```python
from build123d import *

# Parameters (mm, degrees)
SKETCH1_W           = 10
SKETCH1_H           = 5
BOSS_EXTRUDE1_DEPTH = 200
SKETCH2_R           = 2.38125
CUT_EXTRUDE1_DEPTH  = 200


with BuildPart() as part:
    # Sketch1 → Boss-Extrude1 (new body)
    with BuildSketch(Plane.XY):
        with Locations((-10, 62.5)):
            Rectangle(SKETCH1_W, SKETCH1_H)
        with BuildLine():
            Line((90, 0), (60, 0))
            ThreePointArc((60, 0), (17.573593129, 17.573593129), (0, 60))
            Line((0, 60), (0, 65))
            Line((0, 65), (-5, 65))
            Line((-5, 65), (-5, 60))
            ThreePointArc((-5, 60), (14.038059223, 14.038059223), (60, -5))
            Line((60, -5), (90, -5))
            ThreePointArc((90, -5), (135.961940777, 14.038059223), (155, 60))
            Line((155, 60), (155, 65))
            Line((155, 65), (150, 65))
            Line((150, 65), (150, 60))
            ThreePointArc((150, 60), (132.426406871, 17.573593129), (90, 0))
        make_face()
        with Locations((160, 62.5)):
            Rectangle(SKETCH1_W, SKETCH1_H)
    extrude(amount=BOSS_EXTRUDE1_DEPTH)

    # Sketch2 → Cut-Extrude1 (cut)
    with BuildSketch(Plane(origin=(0, 65, 0), x_dir=(1, 0, 0), z_dir=(0, 1, 0))):
        with Locations((-10, -170)):
            Circle(SKETCH2_R)
        with Locations((-10, -30)):
            Circle(SKETCH2_R)
        with Locations((160, -30)):
            Circle(SKETCH2_R)
        with Locations((160, -170)):
            Circle(SKETCH2_R)
    extrude(amount=-CUT_EXTRUDE1_DEPTH, mode=Mode.SUBTRACT)


solid = part.part
```
Part model, mm, in its own coordinate system. A direction names the side the tool comes from. Coordinates: 2 decimals unless noted, no trailing zeros. Write each loop counter-clockwise with the first axis right and the second up, starting at its lowest first coordinate (ties: lowest second). Pieces come first, ordered by that corner, then holes.
Item 1: Probe line 1 (X direction, y = 62.1, z = 170); line 2 (X direction, y = 59, z = 134); line 3 (X direction, y = 6.5, z = 66). List the from-to ranges inside material, lowest first.
Item 2: Slice it at A-A (z = 30). Write the cut outline in (x, y), and give its area (3 significant figures).
Item 3: Pin check, flat tips, straight feed: pin 1 (8 mm diameter, centred on y = 34, z = 20.5, fed in from +X); pin 2 (1.5 mm diameter, centred on y = 48, z = 161, fed in from +X); pin 3 (11 mm diameter, centred on x = 161.5, z = 51.5, fed in from -Y); pin 4 (8 mm diameter, centred on x = 55.5, y = 4, fed in from +Z). Stop position of each tip, or through.
Item 4: Which spindle directions (+Z, -Z, +X, -X, +Y, -Y) get a long thin tool onto all of the face, cutting with end or side? Do faces 1 (the face through (160, 60, 99)), 2 (the face through (-7, 65, 99)), 3 (the face through (0, 62, 99)), 4 (the face through (-10, 60, 99)). Say none if no direction does.
Item 5: Slice it at B-B (x = 160). Write the cut outline in (y, z), and give its area (3 significant figures).
Item 6: Mould opens along Z. For faces 5 (the face through (75, 0, 99)), 6 (the face through (75, -1, 200)), 7 (the face through (-10.31, 62.54, 27.64)) say: released by +Z, released by -Z, zero draft, split by the parting line, or undercut.
Item 7: Slice it at D-D (y = 27). Write the cut outline in (x, z), and give its area (3 significant figures).
Item 8: Slice it at C-C (z = 85.5). Write the cut outline in (x, y), and give its area (3 significant figures).
Results found:
1. line 1: x = -15 to -12.38, -7.62 to 0, 150 to 157.62, 162.38 to 165
1. line 2: x = -4.99 to 0.01, 149.99 to 154.99
1. line 3: x = 23.08 to 32.84, 117.16 to 126.92
2. outline: (-15, 60) - (-12.38, 60) - (-12.38, 65) - (-15, 65) - close; (-7.62, 60) - (-5, 60) arc R65 ccw to (60, -5) - (90, -5) arc R65 ccw to (155, 60) - (157.62, 60) - (157.62, 65) - (150, 65) - (150, 60) arc R60 cw to (90, 0) - (60, 0) arc R60 cw to (0, 60) - (0, 65) - (-7.62, 65) - close; (162.38, 60) - (165, 60) - (165, 65) - (162.38, 65) - close
2. area: 1,230 mm2
3. pin 1: stops at x = 151.16
3. pin 2: stops at x = 154.02
3. pin 3: stops at y = 60
3. pin 4: stops at z = 200
4. face 1: +Z, -Z, +X, -Y
4. face 2: +Z, -Z, +X, -X, +Y
4. face 3: +Z, -Z, +Y
4. face 4: +Z, -Z, -X, -Y
5. outline: (60, 0) - (65, 0) - (65, 27.62) - (60, 27.62) - close; (60, 32.38) - (65, 32.38) - (65, 167.62) - (60, 167.62) - close; (60, 172.38) - (65, 172.38) - (65, 200) - (60, 200) - close
5. area: 952 mm2
6. face 5: zero draft
6. face 6: released by +Z
6. face 7: undercut
7. outline: (4, 0) - (9.89, 0) - (9.89, 200) - (4, 200) - close; (140.11, 0) - (146, 0) - (146, 200) - (140.11, 200) - close
7. area: 2,360 mm2
8. outline: (-15, 60) - (-5, 60) arc R65 ccw to (60, -5) - (90, -5) arc R65 ccw to (155, 60) - (165, 60) - (165, 65) - (150, 65) - (150, 60) arc R60 cw to (90, 0) - (60, 0) arc R60 cw to (0, 60) - (0, 65) - (-15, 65) - close
8. area: 1,280 mm2
